The listing builds one solid part. Answer for the finished solid, in the listing's coordinates (mm). Coordinates: 2 decimals unless noted, no trailing zeros. Loops run counter-clockwise (first coordinate to the right, second up) from the corner with the lowest first, then second, coordinate; pieces in that order, holes last. Notation, with made-up numbers: (33, 37) - (76, 37) arc R18 cw to (76, 72) - close; hole circle Ø9 at (67.25, 52.25). An arc over 180 degrees is marked (long way). Write each question's results on one line, items separated by ' | '. Start each with the question number.
(1) Consider line 1 (Z direction, x = -1, y = 0.25); line 2 (Z direction, x = 0, y = -4.1); line 3 (X direction, y = -4.4, z = 25). Determine where each line is inside the solid, lowest interval first. Write a range as from..to.
(2) Find section C-C on y = 0. Determine the outline of the cut face in (x, z).
(3) Find section A-A on z = -25. Determine the outline of the cut face in (x, y).
(4) Find section B-B on x = 0. Determine the outline of the cut face in (y, z), then the cut area to 3 significant figures.
(5) Find section D-D on z = 25.5. Determine the outline of the cut face in (x, y), then the cut area to 3 significant figures.
(6) Determine the mould class of faces 1 (the flat face through (2.5, 0, 0)), 2 (the cylindrical face through (1.386, 3.782, -24.425)), 3 (the cylindrical face through (1.386, -3.782, -24.425)), 4 (the flat face through (0, -5, 0)) for opening direction X: released by +X, released by -X, zero draft, split by the parting line, or undercut.
from build123d import *

# Parameters (mm, degrees)
SKETCH_1_W               = 60
SKETCH_1_H               = 10
SKETCH_1_R               = 3
EXTRUDE_1_DEPTH          = 2.5
SKETCH_3_R               = 1.5
CUT_EXTRUDE_1_DEPTH      = 6
CUT_EXTRUDE_1_DEPTH_BACK = 6


with BuildPart() as part:
    # 草圖1 → 填料-伸長1 (new body, symmetric)
    with BuildSketch(Plane(origin=(0, 0, 0), x_dir=(0, 0, -1), z_dir=(1, 0, 0))):
        Rectangle(SKETCH_1_W, SKETCH_1_H)
        with Locations((-25, 0)):
            Circle(SKETCH_1_R, mode=Mode.SUBTRACT)
        with Locations((25, 0)):
            Circle(SKETCH_1_R, mode=Mode.SUBTRACT)
    extrude(amount=EXTRUDE_1_DEPTH, both=True)

    # 草圖3 → 除料-伸長1 (cut, two sides)
    with BuildSketch(Plane(origin=(0, 0, 0), x_dir=(1, 0, 0), z_dir=(0, 1, 0))) as cut_extrude_1_sk:
        with Locations((0, 25)):
            Circle(SKETCH_3_R)
        with Locations((0, -25)):
            Circle(SKETCH_3_R)
    extrude(amount=CUT_EXTRUDE_1_DEPTH, mode=Mode.SUBTRACT)
    extrude(cut_extrude_1_sk.sketch, amount=-CUT_EXTRUDE_1_DEPTH_BACK, mode=Mode.SUBTRACT)


solid = part.part
Values:
1) line 1: z = -30..-27.99, -22.01..22.01, 27.99..30 | line 2: z = -30..-26.5, -23.5..23.5, 26.5..30 | line 3: x = -2.5..-1.5, 1.5..2.5
2) outline: (-2.5, -30) - (2.5, -30) - (2.5, -28) - (-2.5, -28) - close; (-2.5, -22) - (2.5, -22) - (2.5, 22) - (-2.5, 22) - close; (-2.5, 28) - (2.5, 28) - (2.5, 30) - (-2.5, 30) - close
3) outline: (-2.5, -5) - (-1.5, -5) - (-1.5, -3) - (-2.5, -3) - close; (-2.5, 3) - (-1.5, 3) - (-1.5, 5) - (-2.5, 5) - close; (1.5, -5) - (2.5, -5) - (2.5, -3) - (1.5, -3) - close; (1.5, 3) - (2.5, 3) - (2.5, 5) - (1.5, 5) - close
4) outline: (-5, -30) - (5, -30) - (5, -26.5) - (2.6, -26.5) arc R3 cw to (-2.6, -26.5) - (-5, -26.5) - close; (-5, -23.5) - (-2.6, -23.5) arc R3 cw to (2.6, -23.5) - (5, -23.5) - (5, 23.5) - (2.6, 23.5) arc R3 cw to (-2.6, 23.5) - (-5, 23.5) - close; (-5, 26.5) - (-2.6, 26.5) arc R3 cw to (2.6, 26.5) - (5, 26.5) - (5, 30) - (-5, 30) - close | area: 518 mm²
5) outline: (-2.5, -5) - (-1.41, -5) - (-1.41, -2.96) - (-2.5, -2.96) - close; (-2.5, 2.96) - (-1.41, 2.96) - (-1.41, 5) - (-2.5, 5) - close; (1.41, -5) - (2.5, -5) - (2.5, -2.96) - (1.41, -2.96) - close; (1.41, 2.96) - (2.5, 2.96) - (2.5, 5) - (1.41, 5) - close | area: 8.87 mm²
6) face 1: released by +X | face 2: undercut | face 3: undercut | face 4: zero draft
